```python
from build123d import *

# Parameters (mm, degrees)
BOSS_EXTRUDE1_DEPTH   = 16
BOSS_EXTRUDE1_2_DEPTH = 16
BOSS_EXTRUDE4_DEPTH   = 5
BOSS_EXTRUDE5_START   = 5
BOSS_EXTRUDE5_DEPTH   = 5
SKETCH7_W             = 20
SKETCH7_H             = 26
SKETCH7_W_2           = 15
SKETCH7_H_2           = 21
BOSS_EXTRUDE6_DEPTH   = 10
SKETCH9_W             = 10
SKETCH9_H             = 34.5
BOSS_EXTRUDE7_DEPTH   = 18
BOSS_EXTRUDE8_DEPTH   = 12
CUT_EXTRUDE3_DEPTH    = 10
SKETCH12_W            = 18
SKETCH12_H            = 6
BOSS_EXTRUDE9_DEPTH   = 18
SKETCH13_R            = 3.125
CUT_EXTRUDE4_DEPTH    = 18


with BuildPart() as part:
    # Sketch1 → Boss-Extrude1 (new body)
    with BuildSketch(Plane.XY):
        with BuildLine():
            Line((-40.982019254, 48.053087066), (1.444387617, 5.626680195))
            ThreePointArc((1.444387617, 5.626680195), (6.46743153, 2.270389555), (12.392515814, 1.091817013))
            Line((12.392515814, 1.091817013), (22.804554858, 1.091817013))
            ThreePointArc((22.804554858, 1.091817013), (26.755839943, -0.544858858), (28.392515814, -4.496143942))
            Line((28.392515814, -4.496143942), (28.392515814, -13.908182987))
            Line((28.392515814, -13.908182987), (33.392515814, -13.908182987))
            Line((33.392515814, -13.908182987), (33.392515814, -4.496143942))
            ThreePointArc((33.392515814, -4.496143942), (30.291373849, 2.990675048), (22.804554858, 6.091817013))
            Line((22.804554858, 6.091817013), (12.392515814, 6.091817013))
            ThreePointArc((12.392515814, 6.091817013), (8.380848692, 6.889787217), (4.979921523, 9.162214101))
            Line((4.979921523, 9.162214101), (-37.446485348, 51.588620972))
            Line((-37.446485348, 51.588620972), (-42.446485348, 51.588620972))
            ThreePointArc((-42.446485348, 51.588620972), (-42.065883011, 49.67520381), (-40.982019254, 48.053087066))
        make_face()
    extrude(amount=BOSS_EXTRUDE1_DEPTH)



with BuildPart() as body_2:
    # Sketch1 → Boss-Extrude1 2 (new body)
    with BuildSketch(Plane.XY):
        with BuildLine():
            Line((-48.053087066, 40.982019254), (-5.626680195, -1.444387617))
            ThreePointArc((-5.626680195, -1.444387617), (2.640597206, -6.96840577), (12.392515814, -8.908182987))
            Line((12.392515814, -8.908182987), (12.392515814, -13.908182987))
            ThreePointArc((12.392515814, -13.908182987), (0.727180044, -11.587803433), (-9.162214101, -4.979921523))
            Line((-9.162214101, -4.979921523), (-51.588620972, 37.446485348))
            ThreePointArc((-51.588620972, 37.446485348), (-55.924075998, 43.934952324), (-57.446485348, 51.588620972))
            Line((-57.446485348, 51.588620972), (-52.446485348, 51.588620972))
            ThreePointArc((-52.446485348, 51.588620972), (-51.304678336, 45.848369486), (-48.053087066, 40.982019254))
        make_face()
    extrude(amount=BOSS_EXTRUDE1_2_DEPTH)


with BuildPart() as part_1:
    add(part.part)

    add(body_2.part)  # Boss-Extrude4 merges body 2
    # Sketch5 → Boss-Extrude4 (add)
    with BuildSketch(Plane.XY.offset(16)):
        with BuildLine():
            Line((-57.446485348, 51.588620972), (-37.446485348, 51.588620972))
            Line((-37.446485348, 51.588620972), (4.979921523, 9.162214101))
            ThreePointArc((4.979921523, 9.162214101), (8.380848692, 6.889787217), (12.392515814, 6.091817013))
            Line((12.392515814, 6.091817013), (22.804554858, 6.091817013))
            ThreePointArc((22.804554858, 6.091817013), (30.291373849, 2.990675048), (33.392515814, -4.496143942))
            Line((33.392515814, -4.496143942), (33.392515814, -13.908182987))
            Line((33.392515814, -13.908182987), (12.392515814, -13.908182987))
            ThreePointArc((12.392515814, -13.908182987), (0.727180044, -11.587803433), (-9.162214101, -4.979921523))
            Line((-9.162214101, -4.979921523), (-51.588620972, 37.446485348))
            ThreePointArc((-51.588620972, 37.446485348), (-55.924075998, 43.934952324), (-57.446485348, 51.588620972))
        make_face()
    extrude(amount=BOSS_EXTRUDE4_DEPTH)

    # Sketch6 → Boss-Extrude5 (add)
    with BuildSketch(Plane(origin=(0, 0, 0), x_dir=(-1, 0, 0), z_dir=(0, 0, -1)).offset(BOSS_EXTRUDE5_START)):
        with BuildLine():
            Line((-4.979921523, 9.162214101), (37.446485348, 51.588620972))
            Line((37.446485348, 51.588620972), (57.446485348, 51.588620972))
            ThreePointArc((57.446485348, 51.588620972), (55.924075998, 43.934952324), (51.588620972, 37.446485348))
            Line((51.588620972, 37.446485348), (9.162214101, -4.979921523))
            ThreePointArc((9.162214101, -4.979921523), (-0.727180044, -11.587803433), (-12.392515814, -13.908182987))
            Line((-12.392515814, -13.908182987), (-33.392515814, -13.908182987))
            Line((-33.392515814, -13.908182987), (-33.392515814, -4.496143942))
            ThreePointArc((-33.392515814, -4.496143942), (-30.291373849, 2.990675048), (-22.804554858, 6.091817013))
            Line((-22.804554858, 6.091817013), (-12.392515814, 6.091817013))
            ThreePointArc((-12.392515814, 6.091817013), (-8.380848692, 6.889787217), (-4.979921523, 9.162214101))
        make_face()
        Polygon((28.607650583, 35.678718395), (10.929981054, 18.001048865), (18.001048865, 10.929981054), (35.678718395, 28.607650583), align=None, mode=Mode.SUBTRACT)
    extrude(amount=-BOSS_EXTRUDE5_DEPTH)

    # Sketch7 → Boss-Extrude6 (add)
    with BuildSketch(Plane(origin=(0, 51.588620972, 0), x_dir=(1, 0, 0), z_dir=(0, 1, 0))):
        with Locations((-47.446485348, -8)):
            Rectangle(SKETCH7_W, SKETCH7_H)
        with Locations((-47.446485348, -8)):
            Rectangle(SKETCH7_W_2, SKETCH7_H_2, mode=Mode.SUBTRACT)
    extrude(amount=BOSS_EXTRUDE6_DEPTH)

    # Sketch9 → Boss-Extrude7 (add)
    with BuildSketch(Plane(origin=(7.071067812, 7.071067812, 0), x_dir=(0, 0, -1), z_dir=(0.7071067811865486, 0.7071067811865465, 0))):
        with Locations((-10, 29.707327442)):
            Rectangle(SKETCH9_W, SKETCH9_H)
    extrude(amount=BOSS_EXTRUDE7_DEPTH)

    # Sketch10 → Boss-Extrude8 (add)
    with BuildSketch(Plane(origin=(0, 0, 5), x_dir=(-1, 0, 0), z_dir=(0, 0, -1))):
        Polygon((20.82947599, 45.578213332), (17.293942084, 42.042679426), (9.869320882, 49.467300628), (13.404854788, 53.002834534), align=None)
        Polygon((-10.990329163, 28.607650583), (-7.454795257, 32.143184489), (-0.030174055, 24.718563287), (-3.565707961, 21.183029381), align=None)
    extrude(amount=BOSS_EXTRUDE8_DEPTH)

    # Sketch11 → Cut-Extrude3 (cut)
    with BuildSketch(Plane(origin=(0, 0, -5), x_dir=(-1, 0, 0), z_dir=(0, 0, -1))):
        Polygon((24.365009896, 31.436077708), (20.82947599, 34.971611614), (16.233281912, 30.375417536), (9.515767491, 23.657903115), (13.051301397, 20.122369209), (19.768815818, 26.83988363), align=None)
    extrude(amount=-CUT_EXTRUDE3_DEPTH, mode=Mode.SUBTRACT)

    # Sketch12 → Boss-Extrude9 (add)
    with BuildSketch(Plane.XY.offset(21)):
        with Locations((-3.233952637, 1.091817013)):
            Rectangle(SKETCH12_W, SKETCH12_H)
    extrude(amount=BOSS_EXTRUDE9_DEPTH)

    # Sketch13 → Cut-Extrude4 (cut)
    with BuildSketch(Plane(origin=(0, 4.091817013, 0), x_dir=(1, 0, 0), z_dir=(0, 1, 0))):
        with Locations(Location((-3.233952637, -30, 0), (0, 0, 270))):
            Circle(SKETCH13_R)
    extrude(amount=-CUT_EXTRUDE4_DEPTH, mode=Mode.SUBTRACT)


solid = part_1.part
```
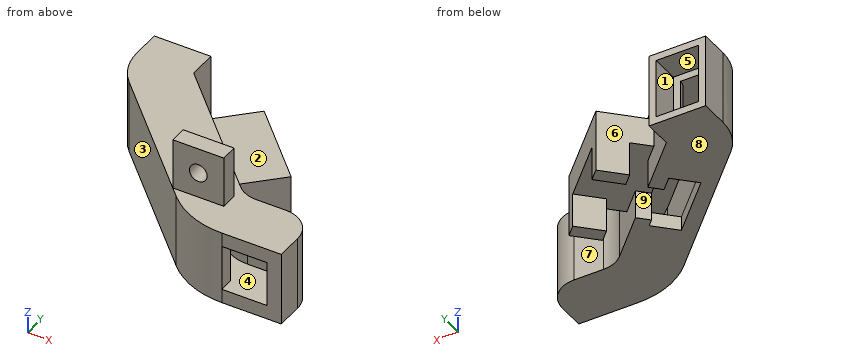
Source: CAD feature listing. Evaluate the final solid. Frame: model axes, mm. Face numbers are marked on the shaded views. A direction names the side the tool comes from. Coordinates: 2 decimals unless noted, no trailing zeros. Loops run counter-clockwise (first coordinate to the right, second up) from the corner with the lowest first, then second, coordinate; pieces in that order, holes last. Notation, with made-up numbers: (64, 66) -> (69, 66) arc R30 ccw to (69, 103) -> close; hole circle Ø9 at (-34, 24.25). An arc over 180 degrees is marked (long way). One line per item, written item: value. Start each with the question number.
Q1. Section query D-D, the plane z = 30. Return the cut outline in (x, y).
Q2. Line query: line 1 along Z through (x, y) = (-10, 14); line 2 along X through (y, z) = (2.7, 30); line 3 along Y through (x, z) = (-3.5, 13). Output: solid intervals per line, ascending.
Q3. Section query C-C, the plane y = 2.5. Return the cut outline in (x, z) (3 decimals).
Q4. Set-up query: the marked faces 5, 6, 7, 8 and 9. Return all of +Z, -Z, +X, -X, +Y, -Y with unobstructed straight access to the full face (end or side cutting, diameter ignored); none if empty.
Q5. Mould query, pull axis Z, two halves, no side actions, for the marked faces 1, 2, 3 and 4. Classes: pulls with the +Z half, pulls with the -Z half, needs draft (parallel to the pull), parting line crosses it, or undercut.
Q6. Section query B-B, the plane x = 16.5. Return the cut outline in (y, z), and give its area (3 significant figures).
Q7. Contact query for flat-ended pins moving along their axis: P1, Ø3, axis at y = 22.5, z = -1, coming from the -X side; P2, Ø11.5, axis at x = -35, y = 44.5, coming from the +Z side; P3, Ø3, axis at y = 2, z = 29, coming from the +X side. Output: stop coordinate, or through.
Results:
1. outline: (-12.23, -1.91) -> (-6.36, -1.91) -> (-6.36, 4.09) -> (-12.23, 4.09) -> close; (-0.11, -1.91) -> (5.77, -1.91) -> (5.77, 4.09) -> (-0.11, 4.09) -> close
2. line 1: -5 to 0, 16 to 21
2. line 2: -12.23 to -6.36, -0.11 to 5.77
2. line 3: -9.44 to -3.35, 10.57 to 43.1
3. outline: (-16.642, -5) -> (30.752, -5) -> (30.752, 21) -> (5.766, 21) -> (5.766, 39) -> (-12.234, 39) -> (-12.234, 21) -> (-16.642, 21) -> close; hole (-9.571, 0) -> (5.941, 0) -> (5.941, 16) -> (-9.571, 16) -> close; hole circle Ø6.25 at (-3.234, 30)
4. face 5: +Y
4. face 6: +Z, -Z, +Y
4. face 7: +Z, -Z, +X, +Y
4. face 8: -Z, -X, -Y
4. face 9: -Z
5. face 1: undercut
5. face 2: pulls with the +Z half
5. face 3: needs draft
5. face 4: undercut
6. outline: (-13.91, -5) -> (6.09, -5) -> (6.09, 21) -> (-13.91, 21) -> (-13.91, 16) -> (1.09, 16) -> (1.09, 0) -> (-13.91, 0) -> close
6. area: 280 mm^2
7. P1: x = -38.14
7. P2: z = 21
7. P3: x = 5.77
